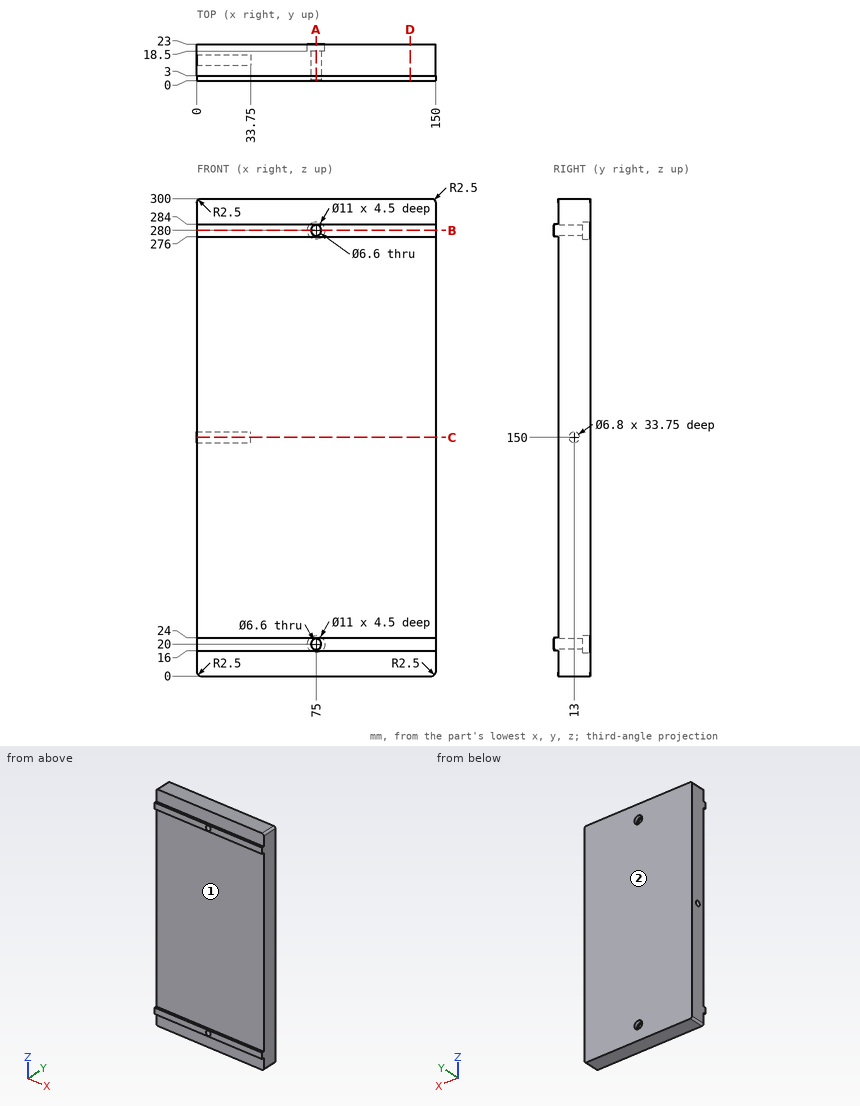
Could you check a few things on this drawing? It's one solid part, dimensions in mm from its lowest x, y, z. Coordinates: 2 decimals unless noted, no trailing zeros. Order: outer loops, then holes, each group sorted by start corner. A loop starts at its lowest first (then second) coordinate and runs counter-clockwise, first axis right, second up. Notation, with made-up numbers: (8.25, 27.5) -> (29.25, 27.5) arc R29 ccw to (29.25, 65.5) -> close; hole circle Ø6 at (17.25, -7). An arc over 180 degrees is marked (long way). Answer in a Markdown table with one row per item.
(1) I want a section at B-B on z = 280. List the corners of the cut face in (x, y) for me, then the cut area to 3 significant figures.
Answer key:
| item | result |
|---|---|
| outline | (0, 0) -> (71.7, 0) -> (71.7, 18.5) -> (69.5, 18.5) -> (69.5, 23) -> (0, 23) -> close; (78.3, 0) -> (150, 0) -> (150, 23) -> (80.5, 23) -> (80.5, 18.5) -> (78.3, 18.5) -> close |
| area | 3,280 mm^2 |
(2) Will these pins go through, and if not, where does the flat tip stop? pin 1 Ø1.5 at (x, y) = (46.5, 2) entering from -Z; pin 2 Ø8 at (x, z) = (88, 288.5) entering from -Y; pin 3 Ø4 at (y, z) = (13, 150) entering from -X.
Answer key:
| item | result |
|---|---|
| pin 1 | z = 16 |
| pin 2 | y = 3 |
| pin 3 | x = 33.75 |
(3) Please list where these lines run through material, in increasing order: probe 1 along Z at (x, y) = (75, 14.5); probe 2 along X at (y, z) = (19.65, 20); probe 3 along Z at (x, y) = (75, 19.65).
Answer key:
| item | result |
|---|---|
| probe 1 | 0 to 16.7, 23.3 to 276.7, 283.3 to 300 |
| probe 2 | 0 to 69.5, 80.5 to 150 |
| probe 3 | 0 to 14.5, 25.5 to 274.5, 285.5 to 300 |
(4) I want a section at C-C on z = 150. List the corners of the cut face in (x, y) for me, then the cut area to 3 significant figures.
Answer key:
| item | result |
|---|---|
| outline | (0, 3) -> (150, 3) -> (150, 23) -> (0, 23) -> (0, 16.4) -> (33.75, 16.4) -> (33.75, 9.6) -> (0, 9.6) -> close |
| area | 2,770 mm^2 |
(5) I want a section at A-A on x = 75. List the corners of the cut face in (y, z) for me.
Answer key:
| item | result |
|---|---|
| outline | (0, 16) -> (3, 16) -> (3, 0) -> (23, 0) -> (23, 14.5) -> (18.5, 14.5) -> (18.5, 16.7) -> (0, 16.7) -> close; (0, 23.3) -> (18.5, 23.3) -> (18.5, 25.5) -> (23, 25.5) -> (23, 274.5) -> (18.5, 274.5) -> (18.5, 276.7) -> (0, 276.7) -> (0, 276) -> (3, 276) -> (3, 24) -> (0, 24) -> close; (0, 283.3) -> (18.5, 283.3) -> (18.5, 285.5) -> (23, 285.5) -> (23, 300) -> (3, 300) -> (3, 284) -> (0, 284) -> close |
(6) Thinking about a two-plate mould opening in Z: for the marked faces 1 and 2, which applies, +Z half, -Z half, draft (parallel to the pull), parting line (faces both ways), or undercut?
Answer key:
| item | result |
|---|---|
| face 1 | undercut |
| face 2 | draft |
(7) I want a section at D-D on x = 134. List the corners of the cut face in (y, z) for me.
Answer key:
| item | result |
|---|---|
| outline | (0, 16) -> (3, 16) -> (3, 0) -> (23, 0) -> (23, 300) -> (3, 300) -> (3, 284) -> (0, 284) -> (0, 276) -> (3, 276) -> (3, 24) -> (0, 24) -> close |
